Part model, mm, in its own coordinate system. Face numbers are marked on the shaded views. A direction names the side the tool comes from. Give positions to 0.01 mm unless a question says otherwise; leave off trailing zeros. Write each loop counter-clockwise with the first axis right and the second up, starting at its lowest first coordinate (ties: lowest second). Pieces come first, ordered by that corner, then holes.
Autodesk Inventor part; units mm, degrees
ref_plane "Work Plane2" through (-18, -67, -25) normal (-1, 0, 0) x (0, 0, 1)
ref_plane "Work Plane3" through (37, -80.7499, -30.1921) normal (-1, 0, 0) x (0, -0.417504, 0.9086751)
ref_plane "Work Plane4" through (37, -71, -27) normal (0, -1, 0) x (1, 0, 0)
ref_plane "Work Plane1" through (-10, 0, 0) normal (0, 0, 1) x (1, 0, 0)
sketch "Sketch1" plane through (-10, 0, 0) normal (0, 0, 1) x (1, 0, 0)
  line L0 (38, 30) -> (40, 28) construction
  line L1 (38, 30) -> (-18, 30) construction
  line L2 (-20, 28) -> (-18, 30) construction
  line L3 (-20, 28) -> (-20, -28) construction
  line L4 (-18, -30) -> (-20, -28) construction
  line L5 (-18, -30) -> (38, -30) construction
  line L6 (40, -28) -> (38, -30) construction
  line L7 (40, -28) -> (40, 28) construction
  circle A0 centre (-7.5, 17.5) radius 1.95 construction
  circle A1 centre (-7.5, -17.5) radius 1.95 construction
  circle A2 centre (27.5, -17.5) radius 1.95 construction
  circle A3 centre (27.5, 17.5) radius 1.95 construction
  circle A4 centre (10, 0) radius 7.5 construction
  circle A5 centre (-5, -51) radius 1 construction
  circle A6 centre (25, -58.5) radius 1 construction
  circle A7 centre (25, -42.5) radius 1.0474 construction
  circle A8 centre (35, -42.5) radius 1 construction
  circle A9 centre (35, -51) radius 1 construction
  circle A10 centre (35, -58.5) radius 1 construction
  circle A11 centre (25, -51) radius 1 construction
  circle A12 centre (-5, -59) radius 1 construction
  circle A13 centre (-5, -43) radius 1 construction
  line L8 (-8, -67) -> (-8, -35) construction
  line L9 (-8, -67) -> (40, -67) construction
  line L10 (40, -35) -> (40, -67) construction
  line L11 (-8, -35) -> (40, -35) construction
  line L12 (38, 30) -> (40, 28)
  line L13 (38, 30) -> (-18, 30)
  line L14 (-20, 28) -> (-18, 30)
  line L15 (-20, 28) -> (-20, -28)
  line L16 (-18, -30) -> (-20, -28)
  line L17 (-18, -30) -> (38, -30)
  line L18 (40, -28) -> (38, -30)
  line L19 (40, -28) -> (40, 28)
  circle A14 centre (-7.5, 17.5) radius 1.95
  circle A15 centre (-7.5, -17.5) radius 1.95
  circle A16 centre (27.5, -17.5) radius 1.95
  circle A17 centre (27.5, 17.5) radius 1.95
  circle A18 centre (10, 0) radius 7.5
  line L20 (-8, -35) -> (40, -35)
  line L21 (-8, -67) -> (-8, -35)
  line L22 (-8, -67) -> (40, -67)
  line L23 (40, -35) -> (40, -67)
  line L24 (-18, -30) -> (-8, -35)
  line L25 (40, -35) -> (40, -28)
  line L26 (40, -67) -> (47, -67)
  line L27 (47, -67) -> (47, -35)
  line L28 (47, -35) -> (40, -35)
  line L29 (40, -35) -> (40, -67)
  line L30 (40, -35) -> (47, -35)
  line L31 (47, -35) -> (47, -25)
  line L32 (47, -25) -> (40, -25)
  line L33 (40, -25) -> (40, -35)
  circle A19 centre (-5, -43) radius 1.5
  circle A20 centre (-5, -51) radius 1.5
  circle A21 centre (-5, -59) radius 1.5
  circle A22 centre (25, -42.5) radius 1.5
  circle A23 centre (25, -51) radius 1.5
  circle A24 centre (25, -58.5) radius 1.5
  circle A25 centre (35, -42.5) radius 1.5
  circle A26 centre (35, -51) radius 1.5
  circle A27 centre (35, -58.5) radius 1.5
  point P0 (10, 0)
extrude "Extrusion1" add sketch "Sketch1" along normal blind 5 contours L12 L19 L18 L17 L16 L15 L14 L13 | L25 L20 L24 L17 L18
sketch "Sketch2" plane through (30, -35, 0) normal (1, 0, 0) x (0, 0, -1)
  line L0 (0, 0) -> (0, 63)
  line L1 (0, 63) -> (-5, 63)
  line L2 (-5, 0) -> (-5, 63)
  line L3 (0, 0) -> (-5, 0)
  circle A0 centre (24, -16) radius 6
  line L4 (8, -32) -> (40, -32)
  line L5 (40, -32) -> (40, 0)
  line L6 (40, 0) -> (8, 0)
  line L7 (8, 0) -> (8, -32)
  line L8 (8, -32) -> (5, -32)
  line L9 (5, -32) -> (5, 0)
  line L10 (5, 0) -> (8, 0)
  line L11 (8, 0) -> (8, -32)
  line L12 (5, 0) -> (-5, 12.3524)
  line L13 (0, 0) -> (-5, 0)
  line L14 (5, 0) -> (-5, 0)
  line L15 (-5, 0) -> (-5, 12.3524)
  point P0 (0, 35)
  dimension "d11" = 3
ref_plane "Work Plane2" through (-18, -67, -25) normal (-1, 0, 0) x (0, 0, 1)
extrude "Extrusion2" add sketch "Sketch2" against normal up to surface (48 mm away) contours L10 L7 L8 L9
sketch "Sketch4" plane through (30, -35, 0) normal (1, 0, 0) x (0, 0, -1)
  line L0 (0, 63) -> (-5, 63)
  line L1 (0, 0) -> (-5, 0)
  line L2 (-5, 0) -> (-5, 63)
  line L3 (0, 0) -> (0, 63)
  point P0 (0, 35)
ref_plane "Work Plane3" through (37, -80.7499, -30.1921) normal (-1, 0, 0) x (0, -0.417504, 0.9086751)
extrude "Extrusion4" add sketch "Sketch4" along normal up to surface (7 mm away)
sketch "Sketch5" plane through (37, -35, 0) normal (1, 0, 0) x (0, 0, -1)
  line L0 (0, 0) -> (-5, 0) construction
  line L1 (8, 0) -> (8, -32) construction
  circle A0 centre (14, -33.5) radius 1 construction
  circle A1 centre (34, -33.5) radius 1 construction
  circle A2 centre (19, -5.5) radius 1 construction
  line L2 (21.4305, -36) -> (8, -36) construction
  line L3 (-5, 0) -> (0, 0)
  line L4 (-5, 0) -> (8, -36)
  line L5 (8, -36) -> (36.2413, -36)
  line L6 (36.2413, -36) -> (36.2413, -25.2619)
  line L7 (36.2413, -25.2619) -> (27.7239, -25.2619)
  line L8 (27.7239, -25.2619) -> (27.7239, 0)
  line L9 (27.7239, 0) -> (0, 0)
  line L10 (0, 0) -> (-5, 0)
  circle A3 centre (24, -16) radius 2.6486 construction
  line L11 (31.5, -8.5) -> (16.5, -8.5)
  line L12 (16.5, -8.5) -> (16.5, -23.5)
  line L13 (16.5, -23.5) -> (31.5, -23.5)
  line L14 (31.5, -23.5) -> (31.5, -8.5)
  line L15 (31.5, -8.5) -> (16.5, -23.5) construction
  line L16 (16.5, -8.5) -> (31.5, -23.5) construction
  circle A4 centre (34.5, -27) radius 1 construction
  line L17 (27.7239, 0) -> (36.2413, 0)
  line L18 (36.2413, 0) -> (36.2413, -7.9172)
  line L19 (36.2413, -7.9172) -> (27.7239, -7.9172)
  line L20 (27.7239, -7.9172) -> (27.7239, 0)
  point P0 (0, 35)
  point P1 (27.7239, -23.5)
  point P2 (27.7239, -8.5)
  dimension "d38" = 15
  dimension "d39" = 15
extrude "Extrusion5" add sketch "Sketch5" against normal blind 3 contours L3 L9 L8 L11 L12 L13 L7 L6 L5 L4 | L17 L18 L19 L8
ref_plane "Work Plane4" through (37, -71, -27) normal (0, -1, 0) x (1, 0, 0)
sketch "Sketch8" plane through (37, 28, 5) normal (1, 0, 0) x (0, 0, -1)
  circle A0 centre (19, -96.5) radius 1
  line L0 (16, -99) -> (41.7, -99)
  circle A1 centre (39.5, -90) radius 1
  circle A2 centre (24, -68.5) radius 1
  point P0 (5, -28)
extrude "Extrusion8" cut sketch "Sketch8" against normal through all
sketch "Sketch9" plane through (-18, -67, -5) normal (-1, 0, 0) x (0, 0, 1)
  line L0 (-3, 0) -> (0, 0) construction
  line L1 (0, 0) -> (0, 32) construction
  line L2 (-3, 0) -> (-3, 32) construction
  line L3 (0, 32) -> (-3, 32) construction
  line L4 (-3, 0) -> (10, 32) construction
  line L5 (5, 32) -> (10, 32) construction
  line L6 (10, 32) -> (0, 32) construction
  line L7 (0, 32) -> (10, 32)
  line L8 (10, 32) -> (10, 0)
  line L9 (10, 0) -> (0, 0)
  line L10 (0, 0) -> (0, 32)
  line L11 (-3, 32) -> (0, 32)
  line L12 (0, 32) -> (0, 0)
  line L13 (0, 0) -> (-3, 0)
  line L14 (-3, 0) -> (-3, 32)
  point P0 (5, 67)
extrude "Extrusion9" add sketch "Sketch9" against normal up to surface (55 mm away)
sketch "Sketch11" plane through (-10, 0, 5) normal (0, 0, 1) x (1, 0, 0)
  circle A0 centre (10, 0) radius 7.5
  circle A1 centre (27.5, 17.5) radius 1.95
  circle A2 centre (27.5, -17.5) radius 1.95
  circle A3 centre (-7.5, -17.5) radius 1.95
  circle A4 centre (-7.5, 17.5) radius 1.95
  line L0 (-18, -30) -> (-8, -35)
  line L1 (-8, -67) -> (-8, -35)
  line L2 (-8, -67) -> (47, -67)
  line L3 (47, 28) -> (47, -67)
  line L4 (40, 28) -> (47, 28)
  line L5 (40, 28) -> (38, 30)
  line L6 (38, 30) -> (-18, 30)
  line L7 (-18, 30) -> (-20, 28)
  line L8 (-20, 28) -> (-20, -28)
  line L9 (-20, -28) -> (-18, -30)
  point P0 (10, 0)
extrude "Extrusion11" [suppressed]
sketch "Sketch12" plane through (37, -35, 0) normal (1, 0, 0) x (0, 0, -1)
  circle A0 centre (19, -5.5) radius 1
  circle A1 centre (14, -33.5) radius 1
  circle A2 centre (34.5, -27) radius 1
  line L0 (0, 0) -> (0, 63)
  line L1 (0, 63) -> (-5, 63)
  line L2 (-5, -32) -> (6.5556, -32)
  line L3 (6.5556, -32) -> (8, -36)
  line L4 (8, -36) -> (36.2413, -36)
  line L5 (36.2413, -36) -> (36.2413, -25.2619)
  line L6 (36.2413, -25.2619) -> (27.7239, -25.2619)
  line L7 (27.7239, -25.2619) -> (27.7239, -23.5)
  line L8 (27.7239, -23.5) -> (16.5, -23.5)
  line L9 (16.5, -23.5) -> (16.5, -8.5)
  line L10 (16.5, -8.5) -> (27.7239, -8.5)
  line L11 (27.7239, -8.5) -> (27.7239, -7.9172)
  line L12 (27.7239, -7.9172) -> (36.2413, -7.9172)
  line L13 (36.2413, -7.9172) -> (36.2413, 0)
  line L14 (36.2413, 0) -> (0, 0)
  line L15 (-5, 63) -> (-5, -32)
  point P0 (0, 35)
extrude "Extrusion12" add sketch "Sketch12" along normal blind 2
sketch "Sketch13" plane through (-18, -67, -8) normal (-1, 0, 0) x (0, 0, 1)
  line L0 (0, 0) -> (13, 0)
  line L1 (8, 32) -> (13, 32)
  line L2 (8, 32) -> (0, 32)
  line L3 (0, 32) -> (0, 0)
  line L4 (8, 39) -> (13, 39)
  line L5 (8, 32) -> (15, 32)
  line L6 (8, 39) -> (8, 32)
  line L7 (8, 32) -> (15, 32)
  line L8 (13, 0) -> (13, 32)
  line L9 (8, 32) -> (13, 32)
  line L10 (13, 32) -> (13, 39)
  line L11 (13, 39) -> (8, 39)
  line L12 (8, 39) -> (8, 32)
  point P0 (8, 67)
ref_plane "Work Plane5" through (-29, -67, -40) normal (-1, 0, 0) x (0, 0, 1)
extrude "Extrusion13" add sketch "Sketch13" along normal up to surface (12 mm away)
sketch "Sketch14" plane through (-10, 0, 5) normal (0, 0, 1) x (1, 0, 0)
  circle A0 centre (14, -43.5) radius 1 construction
  circle A1 centre (24, -43.5) radius 1 construction
  circle A2 centre (-16, -43) radius 1 construction
  circle A3 centre (-16, -59) radius 1 construction
  circle A4 centre (14, -51) radius 1 construction
  circle A5 centre (24, -51) radius 1 construction
  circle A6 centre (24, -59.5) radius 1 construction
  circle A7 centre (14, -59.5) radius 1.0474 construction
  circle A8 centre (-16, -51) radius 1 construction
  line L0 (-19, -35) -> (-19, -67) construction
  line L1 (-19, -35) -> (29, -35) construction
  line L2 (29, -67) -> (29, -35) construction
  line L3 (-19, -67) -> (29, -67) construction
  point P0 (10, 0)
hole "Hole1" at (14, -43.5, 5) at (14, -51, 5) at (14, -59.5, 5) at (4, -59.5, 5) at (4, -51, 5) at (4, -43.5, 5) at (-26, -43, 5) at (-26, -51, 5) at (-26, -59, 5) direction (0, 0, -1) diameter 3.5 depth 16 tip angle 118 counterbore diameter 7 counterbore depth 10
properties part number "10_Adapter_Laser_XY_left"
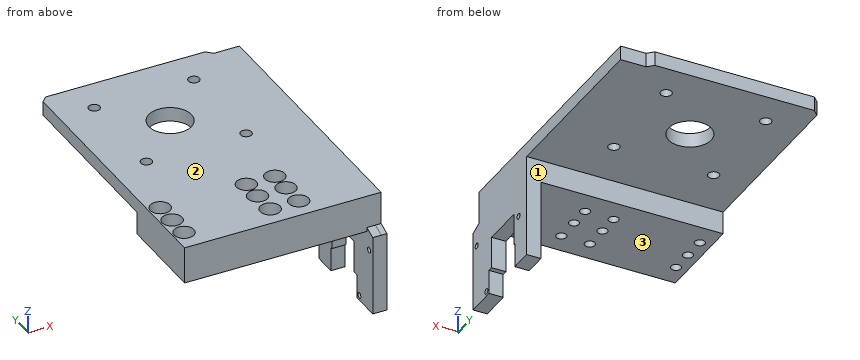
1) Drill centre lines: L1, parallel to Y at x = -26, z = -2; L2, parallel to Y at x = 14, z = -6; L3, parallel to Y at x = 36.15, z = -14. Where is each one in solid material? Low to high.
Check result:
L1: y = -67 to -62.5, -55.5 to -54.5, -47.5 to -46.5, -39.5 to -35
L2: y = -67 to -61.25, -57.75 to -52.75, -49.25 to -45.25, -41.75 to -35
L3: y = -71 to -69.5, -67.5 to -35
2) Saw through at D-D (y = 0). Write the cut outline in (x, z).
Check result:
outline: (-30, 0) - (-7.5, 0) - (-7.5, 5) - (-30, 5) - close; (7.5, 0) - (39, 0) - (39, 5) - (7.5, 5) - close
3) 3-axis set-ups, long thin cutter, end or side, ignore diameter. For the marked faces 1, 2 and 3: which of +Z, -Z, +X, -X, +Y, -Y reach the whole face in a straight line?
Check result:
face 1: -Z, +X, -X, +Y
face 2: +Z, +X, -X, +Y, -Y
face 3: -Z, -X, +Y, -Y
4) Flat gauge pins, fed straight in: P1, Ø3, axis at y = -62, z = -34.5, coming from the +X side; P2, Ø1, axis at x = 11.5, y = -50, coming from the +Z side; P3, Ø4.5, axis at x = 17.5, y = 17.5, coming from the -Z side; P4, Ø5.5, axis at x = 37, z = -21.5, coming from the +Y side. Where does each tip first touch, or does it go through?
Check result:
P1: stops at x = 39
P2: stops at z = -5
P3: stops at z = 0
P4: stops at y = -35
5) Saw through at B-B (z = -22). Write the cut outline in (x, y), and give its area (3 significant figures).
Check result:
outline: (34, -71) - (39, -71) - (39, -58.5) - (34, -58.5) - close; (34, -43.5) - (39, -43.5) - (39, -35) - (34, -35) - close
area: 105 mm2
6) Saw through at C-C (y = -51). State how many separate pieces and enclosed holes the cut face has, and give its area (3 significant figures).
Check result:
separate pieces: 4
enclosed holes: 0
area: 698 mm2
7) Saw through at A-A (y = 17.5). Write the cut outline in (x, z).
Check result:
outline: (-30, 0) - (-19.45, 0) - (-19.45, 5) - (-30, 5) - close; (-15.55, 0) - (15.55, 0) - (15.55, 5) - (-15.55, 5) - close; (19.45, 0) - (39, 0) - (39, 5) - (19.45, 5) - close
